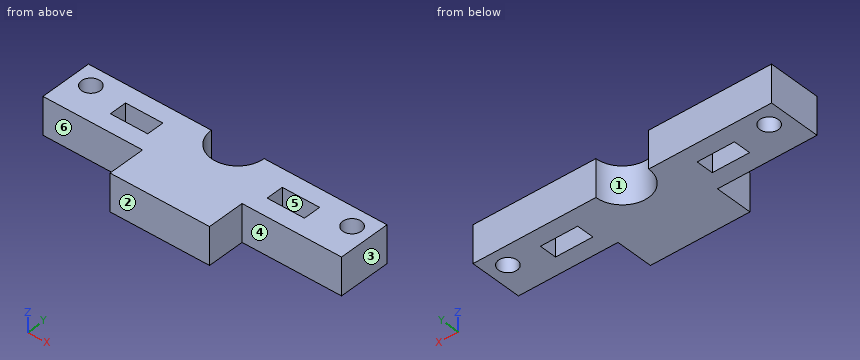
```python
from build123d import *

# Parameters (mm, degrees)
BOSS_EXTRUDE1_DEPTH = 6.35
SKETCH2_R           = 1.5875
CUT_EXTRUDE1_DEPTH  = 53.694769397
SKETCH3_R           = 4.48798261
CUT_EXTRUDE2_DEPTH  = 53.694769397
CAVITY1_START       = 6.554367816
CAVITY1_OUTLINE_W   = 6.35
CAVITY1_OUTLINE_H   = 6.35
CAVITY1_DEPTH       = 2.963333333


# Read off the part's stored shape, not the designer's step: Cavity1
with BuildPart() as part:
    # Sketch1 → Boss-Extrude1 (new body)
    with BuildSketch(Plane.XY):
        Polygon((16.933333333, -2.758965517), (33.866666667, -2.758965517), (33.866666667, 3.591034483), (50.8, 3.591034483), (50.8, 12.481034483), (0, 12.481034483), (0, 3.591034483), (16.933333333, 3.591034483), align=None)
    extrude(amount=BOSS_EXTRUDE1_DEPTH)

    # Sketch2 → Cut-Extrude1 (cut, through all)
    with BuildSketch(Plane(origin=(0, 0, 0), x_dir=(-1, 0, 0), z_dir=(0, 0, -1))):
        with Locations((-47.625, 9.306034483)):
            Circle(SKETCH2_R)
        with Locations((-3.175, 9.306034483)):
            Circle(SKETCH2_R)
    extrude(amount=-CUT_EXTRUDE1_DEPTH, mode=Mode.SUBTRACT)

    # Sketch3 → Cut-Extrude2 (cut, through all)
    with BuildSketch(Plane(origin=(0, 0, 0), x_dir=(-1, 0, 0), z_dir=(0, 0, -1))):
        with Locations((-25.4, 12.481034483)):
            Circle(SKETCH3_R)
    extrude(amount=-CUT_EXTRUDE2_DEPTH, mode=Mode.SUBTRACT)

    # Cavity1 outline → Cavity1 (cut)
    with BuildSketch(Plane(origin=(0, 0, 0), x_dir=(1, 0, 0), z_dir=(0, 1, 0)).offset(CAVITY1_START)):
        with Locations((38.735, -3.175)):
            Rectangle(CAVITY1_OUTLINE_W, CAVITY1_OUTLINE_H)
        with Locations((12.065, -3.175)):
            Rectangle(CAVITY1_OUTLINE_W, CAVITY1_OUTLINE_H)
    extrude(amount=CAVITY1_DEPTH, mode=Mode.SUBTRACT)


solid = part.part
```
Can you work these out from the model? Positions are in its coordinate system, mm. Face numbers are marked on the shaded views. A direction names the side the tool comes from. Coordinates: 2 decimals unless noted, no trailing zeros. Order: outer loops, then holes, each group sorted by start corner. A loop starts at its lowest first (then second) coordinate and runs counter-clockwise, first axis right, second up. Notation, with made-up numbers: (10.25, 64) - (17.25, 64) arc R33 ccw to (17.25, 100) - close; hole circle Ø5 at (53, 77.5). An arc over 180 degrees is marked (long way). Answer in a Markdown table with one row per item.
1. For pin 1 (5 mm diameter, centred on x = 3.18, y = 9.31, fed in from +Z); pin 2 (3 mm diameter, centred on y = 0, z = 3.5, fed in from -X); pin 3 (2.5 mm diameter, centred on x = 47.62, y = 9.31, fed in from +Z); pin 4 (3 mm diameter, centred on x = 41.5, z = 2.5, fed in from -Y), each with a flat end and sliding along its axis, tell me the tip position at first contact or that it passes through.
Reply:
| item | result |
|---|---|
| pin 1 | stops at z = 6.35 |
| pin 2 | stops at x = 16.93 |
| pin 3 | passes through |
| pin 4 | stops at y = 3.59 |
2. If we mould it in two halves opening along X, with no side actions, what happens to the marked faces 1, 2 and 3? For each: pulls with the +X half, pulls with the -X half, needs draft (parallel to the pull), parting line crosses it, or undercut.
Reply:
| item | result |
|---|---|
| face 1 | undercut |
| face 2 | needs draft |
| face 3 | pulls with the +X half |
3. Suppose I cut it at B-B (y = 10). Please give me the cut outline in (x, z).
Reply:
| item | result |
|---|---|
| outline | (0, 0) - (1.75, 0) - (1.75, 6.35) - (0, 6.35) - close; (4.6, 0) - (21.66, 0) - (21.66, 6.35) - (4.6, 6.35) - close; (29.14, 0) - (46.2, 0) - (46.2, 6.35) - (29.14, 6.35) - close; (49.05, 0) - (50.8, 0) - (50.8, 6.35) - (49.05, 6.35) - close |
4. Suppose I cut it at C-C (z = 2.25). Please give me the cut outline in (x, y) (1 decimal), and give its area (3 significant figures).
Reply:
| item | result |
|---|---|
| outline | (0, 3.6) - (16.9, 3.6) - (16.9, -2.8) - (33.9, -2.8) - (33.9, 3.6) - (50.8, 3.6) - (50.8, 12.5) - (29.9, 12.5) arc R4.5 cw to (20.9, 12.5) - (0, 12.5) - close; hole circle Ø3.2 at (3.2, 9.3); hole (8.9, 6.6) - (15.2, 6.6) - (15.2, 9.5) - (8.9, 9.5) - close; hole (35.6, 6.6) - (41.9, 6.6) - (41.9, 9.5) - (35.6, 9.5) - close; hole circle Ø3.2 at (47.6, 9.3) |
| area | 474 mm^2 |
5. Suppose I cut it at A-A (x = 12). Please give me the cut outline in (y, z), and give its area (3 significant figures).
Reply:
| item | result |
|---|---|
| outline | (3.59, 0) - (6.55, 0) - (6.55, 6.35) - (3.59, 6.35) - close; (9.52, 0) - (12.48, 0) - (12.48, 6.35) - (9.52, 6.35) - close |
| area | 37.6 mm^2 |
6. Suppose I cut it at D-D (x = 25.4). Please give me the cut outline in (y, z).
Reply:
| item | result |
|---|---|
| outline | (-2.76, 0) - (7.99, 0) - (7.99, 6.35) - (-2.76, 6.35) - close |
7. For the marked faces 4, 5 and 6, which set-ups out of +Z, -Z, +X, -X, +Y, -Y let a thin tool reach every point of the face, with its end or its side?
Reply:
| item | result |
|---|---|
| face 4 | +Z, -Z, +X, -Y |
| face 5 | +Z, -Z |
| face 6 | +Z, -Z, -X, -Y |
8. If I drill on line 1 along Y through (x, z) = (37.5, 4.5); line 2 along Y through (x, z) = (45.5, 6.25); line 3 along X through (y, z) = (9.75, 5.75), over which ranges is the centre line in solid material (lowest first)?
Reply:
| item | result |
|---|---|
| line 1 | y = 3.59 to 6.55, 9.52 to 12.48 |
| line 2 | y = 3.59 to 12.48 |
| line 3 | x = 0 to 1.65, 4.7 to 21.84, 28.96 to 46.1, 49.15 to 50.8 |
